Geometry check sheet. Reference: the model listing, model coordinates, mm. Face numbers are marked on the shaded views. A direction names the side the tool comes from. Coordinates: 2 decimals unless noted, no trailing zeros. Write each loop counter-clockwise with the first axis right and the second up, starting at its lowest first coordinate (ties: lowest second). Pieces come first, ordered by that corner, then holes. Notation, with made-up numbers: (-11, 10) -> (8, 10) arc R25 ccw to (8, 41) -> close; hole circle Ø3 at (78, 22.25). An arc over 180 degrees is marked (long way). Use a Markdown table: item, result.
```python
from build123d import *

# Parameters (mm, degrees)
REVOLVE1_ANGLE          = 360
CUT_EXTRUDE2_REACH      = 116.3
SKETCH4_W               = 12.7
SKETCH4_H               = 18.796
SKETCH5_R               = 3.3782
CUT_EXTRUDE3_DEPTH      = 31.226
SKETCH6_R               = 1.905
BOSS_EXTRUDE1_DEPTH     = 5.08
SKETCH7_W               = 25.4
SKETCH7_H               = 5.08
BOSS_EXTRUDE4_DEPTH     = 31.75
FILLET1_R               = 6.35
SKETCH8_R               = 3.2639
CUT_EXTRUDE4_DEPTH      = 14.97
CUT_EXTRUDE4_DEPTH_BACK = 101.33


with BuildPart() as part:
    # Sketch1 → Revolve1 (revolve, symmetric)
    with BuildSketch(Plane.XY) as revolve1_sk:
        Polygon((0, 0), (57.15, 0), (57.15, 30.226), (51.816, 30.226), (51.816, 11.43), (0, 11.43), align=None)
    revolve(axis=Axis((0, 0, 0), (0, 1, 0)), revolution_arc=REVOLVE1_ANGLE / 2)
    revolve(revolve1_sk.sketch, axis=Axis((0, 0, 0), (0, -1, 0)), revolution_arc=REVOLVE1_ANGLE / 2)

    # Sketch4 → Cut-Extrude2 (cut, up to next)
    with BuildSketch(Plane(origin=(57.15, 0, 0), x_dir=(0, 0, -1), z_dir=(1, 0, 0)), mode=Mode.PRIVATE) as cut_extrude2_sk1:
        with Locations((0, 20.828)):
            Rectangle(SKETCH4_W, SKETCH4_H)
    cut_extrude2_tool1 = extrude(cut_extrude2_sk1.sketch, amount=-CUT_EXTRUDE2_REACH, mode=Mode.PRIVATE) & part.part
    add(cut_extrude2_tool1.solids().sort_by_distance((57.15, 20.828, 0))[0], mode=Mode.SUBTRACT)

    # Sketch5 → Cut-Extrude3 (cut, through all)
    with BuildSketch(Plane.XZ):
        Circle(SKETCH5_R)
    extrude(amount=-CUT_EXTRUDE3_DEPTH, mode=Mode.SUBTRACT)

    # Sketch6 → Boss-Extrude1 (add)
    with BuildSketch(Plane(origin=(0, 11.43, 0), x_dir=(1, 0, 0), z_dir=(0, 1, 0))):
        with Locations((0, 44.45)):
            Circle(SKETCH6_R)
        with Locations((0, -44.45)):
            Circle(SKETCH6_R)
    extrude(amount=BOSS_EXTRUDE1_DEPTH)

    # Sketch7 → Boss-Extrude4 (add)
    with BuildSketch(Plane(origin=(0, 0, 0), x_dir=(1, 0, 0), z_dir=(0, 1, 0))):
        with Locations((0, -40.64)):
            Rectangle(SKETCH7_W, SKETCH7_H)
        with Locations((0, 40.64)):
            Rectangle(SKETCH7_W, SKETCH7_H)
    extrude(amount=-BOSS_EXTRUDE4_DEPTH)

    # Fillet1
    fillet1_edges = [part.edges().sort_by_distance(p)[0] for p in [
        (12.7, 0, 40.64),
        (-12.7, 0, 40.64),
        (0, 0, 43.18),
        (-12.7, 0, -40.64),
        (12.7, 0, -40.64),
        (0, 0, -43.18),
    ]]
    fillet(fillet1_edges, radius=FILLET1_R)

    # Sketch8 → Cut-Extrude4 (cut, two sides)
    with BuildSketch(Plane.XY.offset(43.18)) as cut_extrude4_sk:
        with Locations((0, -22.225)):
            Circle(SKETCH8_R)
    extrude(amount=CUT_EXTRUDE4_DEPTH, mode=Mode.SUBTRACT)
    extrude(cut_extrude4_sk.sketch, amount=-CUT_EXTRUDE4_DEPTH_BACK, mode=Mode.SUBTRACT)


solid = part.part
```
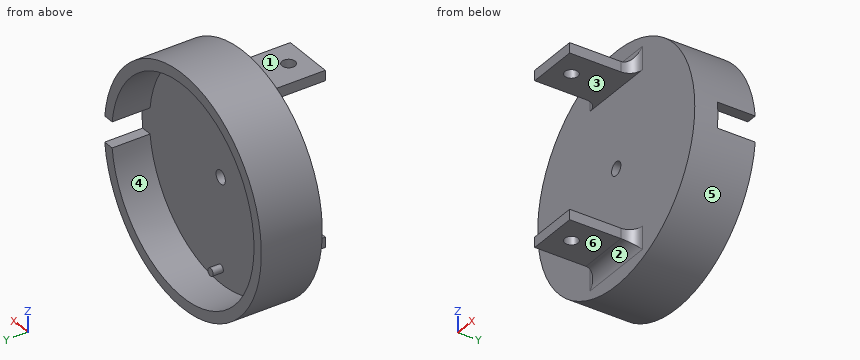
Item 1: Depth check by flat-ended pin: P1, Ø5.5, axis at y = -16, z = -41.5, coming from the -X side; P2, Ø12, axis at y = -20.5, z = 37, coming from the +X side; P3, Ø10.5, axis at x = 0, y = -22.225, coming from the +Z side; P4, Ø4, axis at x = 0, y = -22.225, coming from the +Z side (1 decimal). Enter the tip coordinate at first touch or a pass-through.
Answer block:
| item | result |
|---|---|
| P1 | stops at x = -12.7 |
| P2 | stops at x = 12.7 |
| P3 | stops at z = 43.18 |
| P4 | passes through |
Item 2: Section check A-A on z = 0. Record the boundary of the cut face in (x, y).
Answer block:
| item | result |
|---|---|
| outline | (-57.15, 0) -> (-3.38, 0) -> (-3.38, 11.43) -> (-51.82, 11.43) -> (-51.82, 30.23) -> (-57.15, 30.23) -> close; (3.38, 0) -> (57.15, 0) -> (57.15, 11.43) -> (3.38, 11.43) -> close |
Item 3: Section check D-D on x = 0. Count the separate pieces of the cut face and the enclosed holes in it, then the cut area to 3 significant figures.
Answer block:
| item | result |
|---|---|
| separate pieces | 4 |
| enclosed holes | 0 |
| area | 1,740 mm^2 |
Item 4: Thickness scan on L1, parallel to Z at x = 0, y = 5; L2, parallel to Z at x = 11, y = -14; L3, parallel to Y at x = 37.5, z = 41. Record the ranges inside material, lowest first. Write a range as [from, to].
Answer block:
| item | result |
|---|---|
| L1 | z = [-57.15, -3.38], [3.38, 57.15] |
| L2 | z = [-43.18, -38.1], [38.1, 43.18] |
| L3 | y = [0, 30.23] |
Item 5: Tool access check on the marked faces 1, 2 and 3. Record the directions out of +Z, -Z, +X, -X, +Y, -Y that give a thin tool (end or side, any length) a straight path to the whole face; none if there is none.
Answer block:
| item | result |
|---|---|
| face 1 | +Z, +X, -X, -Y |
| face 2 | -Z, +X, -X, -Y |
| face 3 | +X, -X, -Y |
Item 6: Section check B-B on y = 14. Record the boundary of the cut face in (x, z) (3 decimals), then the cut area to 3 significant figures.
Answer block:
| item | result |
|---|---|
| outline | circle Ø3.81 at (0, -44.45); circle Ø3.81 at (0, 44.45); (51.425, -6.35) arc R51.816 cw (long way) to (51.425, 6.35) -> (56.796, 6.35) arc R57.15 ccw (long way) to (56.796, -6.35) -> close |
| area | 1,780 mm^2 |
Item 7: Section check C-C on x = 24.5. Record the boundary of the cut face in (y, z), then the cut area to 3 significant figures.
Answer block:
| item | result |
|---|---|
| outline | (0, -51.63) -> (30.23, -51.63) -> (30.23, -45.66) -> (11.43, -45.66) -> (11.43, 45.66) -> (30.23, 45.66) -> (30.23, 51.63) -> (0, 51.63) -> close |
| area | 1,400 mm^2 |
Item 8: Mould release check, pull along X, two halves, no side actions. Record for the marked faces 4, 5 and 6: +X half, -X half, draft (parallel to the pull), parting line (faces both ways), or undercut.
Answer block:
| item | result |
|---|---|
| face 4 | undercut |
| face 5 | parting line |
| face 6 | draft |
